Part model, mm, in its own coordinate system. Face numbers are marked on the shaded views. A direction names the side the tool comes from. Coordinates: 2 decimals unless noted, no trailing zeros. Loops run counter-clockwise (first coordinate to the right, second up) from the corner with the lowest first, then second, coordinate; pieces in that order, holes last. Notation, with made-up numbers: (56, 86) -> (80, 86) arc R16 ccw to (80, 97) -> close; hole circle Ø9 at (39.25, -34.5). An arc over 180 degrees is marked (long way). One line per item, written item: value. Start each with the question number.
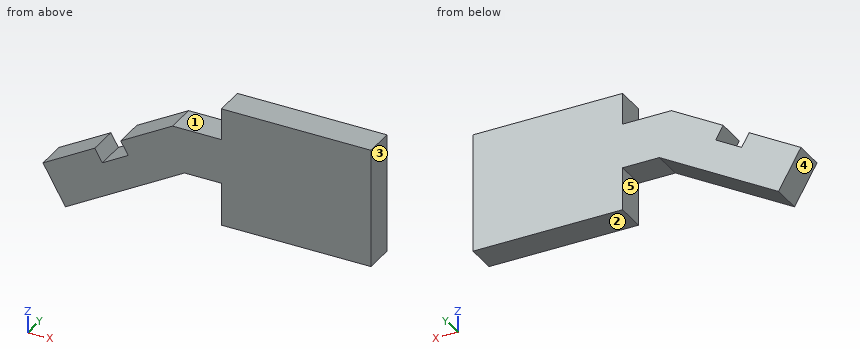
from build123d import *

# Parameters (mm, degrees)
F1_DEPTH = 30


with BuildPart() as f1:
    # F0 (on Front) → F1 (new body)
    with BuildSketch(Plane.XZ):
        Polygon((-54.514028, 15.14498), (-106.475553, -14.85502), (-83.975553, -53.826163), (35.485972, 15.14498), (72.409391, 15.14498), (143.428258, 15.14498), (143.428258, 60.14498), (72.409391, 60.14498), (23.428258, 60.14498), (-28.533266, 30.14498), (-21.033266, 17.154599), (-47.014028, 2.154599), align=None)
        Polygon((143.428258, 15.14498), (72.409391, 15.14498), (72.409391, -28.122669), (222.409391, -28.122669), (222.409391, 91.877331), (72.409391, 91.877331), (72.409391, 84.429644), (72.409391, 60.14498), (143.428258, 60.14498), align=None)
    extrude(amount=F1_DEPTH)


solid = f1.part
1) Slice it at A-A (z = -4). Give the cut face in (x, y).
2) Slice it at D-D (z = 49.5). Give the cut face in (x, y), then the cut area to 3 significant figures.
3) Slice it at B-B (y = -21.25). Give the cut face in (x, z), then the cut area to 3 significant figures.
4) Slice it at C-C (x = 58.5). Give the cut face in (y, z), then the cut area to 3 significant figures.
5) Pin check, flat tips, straight feed: pin 1 Ø9 at (x, y) = (162, -13) entering from -Z; pin 2 Ø4 at (x, y) = (10.5, -10.5) entering from +Z; pin 3 Ø4 at (y, z) = (-10, 51.5) entering from -X. Stop position of each tip, or through.
6) Probe line 1 (X direction, y = -13.75, z = -6); line 2 (X direction, y = -22, z = 34.5); line 3 (X direction, y = -10.75, z = -20). List the from-to ranges inside material, lowest first. Write a range as from..to.
7) Tool access for the marked faces 1, 2, 3, 4 and 5: list every direction of +Z, -Z, +X, -X, +Y, -Y with a clear straight run to the whole face (end or side of a thin tool).
Check sheet entries:
1. outline: (-87.67, -30) -> (2.33, -30) -> (2.33, 0) -> (-87.67, 0) -> close; (72.41, -30) -> (222.41, -30) -> (222.41, 0) -> (72.41, 0) -> close
2. outline: (4.99, -30) -> (222.41, -30) -> (222.41, 0) -> (4.99, 0) -> close
2. area: 6,520 mm^2
3. outline: (-106.48, -14.86) -> (-83.98, -53.83) -> (35.49, 15.14) -> (72.41, 15.14) -> (72.41, -28.12) -> (222.41, -28.12) -> (222.41, 91.88) -> (72.41, 91.88) -> (72.41, 60.14) -> (23.43, 60.14) -> (-28.53, 30.14) -> (-21.03, 17.15) -> (-47.01, 2.15) -> (-54.51, 15.14) -> close
3. area: 26,000 mm^2
4. outline: (-30, 15.14) -> (0, 15.14) -> (0, 60.14) -> (-30, 60.14) -> close
4. area: 1,350 mm^2
5. pin 1: stops at z = -28.12
5. pin 2: stops at z = 53.84
5. pin 3: stops at x = 4.99
6. line 1: x = -91.14..-1.14, 72.41..222.41
6. line 2: x = -20.99..222.41
6. line 3: x = -103.51..-25.39, 72.41..222.41
7. face 1: +Z, -X, +Y, -Y
7. face 2: -Z, +X, +Y, -Y
7. face 3: +Z, -Z, +X, +Y, -Y
7. face 4: -Z, -X, +Y, -Y
7. face 5: -Z, +Y, -Y
